from build123d import *

# Parameters (mm, degrees)
BOSS_EXTRUDE1_DEPTH     = 4
SKETCH3_W               = 9
SKETCH3_H               = 19
SKETCH3_W_2             = 19
SKETCH3_H_2             = 9
BOSS_EXTRUDE2_DEPTH     = 1
CHAMFER1_SIZE           = 1
CUT_EXTRUDE1_DEPTH      = 86
CUT_EXTRUDE1_DEPTH_BACK = 86
SKETCH2_R               = 2.5


with BuildPart() as part:
    # Sketch1 → Boss-Extrude1 (new body)
    with BuildSketch(Plane(origin=(0, 0, 0), x_dir=(1, 0, 0), z_dir=(0, 1, 0))):
        Polygon((0, 0), (0, 60), (20, 60), (60, 20), (60, 0), align=None)
    extrude(amount=BOSS_EXTRUDE1_DEPTH)

    # Sketch3 → Boss-Extrude2 (add)
    with BuildSketch(Plane(origin=(0, 4, 0), x_dir=(1, 0, 0), z_dir=(0, 1, 0))):
        with Locations((10, 50.5)):
            Rectangle(SKETCH3_W, SKETCH3_H)
        with Locations((50.5, 10)):
            Rectangle(SKETCH3_W_2, SKETCH3_H_2)
    extrude(amount=BOSS_EXTRUDE2_DEPTH)

    # Chamfer1
    chamfer1_edges = [part.edges().sort_by_distance(p)[0] for p in [
        (50.5, 5, -14.5),
        (50.5, 5, -5.5),
        (14.5, 5, -50.5),
        (5.5, 5, -50.5),
    ]]
    chamfer(chamfer1_edges, length=CHAMFER1_SIZE - 0.0001)  # a hair under: the kernel refuses the full size

    # Sketch2 → Cut-Extrude1 (cut, two sides: drawn at the far end of the back side and taken through both)
    with BuildSketch(Plane.XZ.offset(-CUT_EXTRUDE1_DEPTH_BACK)):
        with Locations(Location((50, -10, 0), (0, 0, 270))):
            Circle(SKETCH2_R)
        with Locations(Location((30, -10, 0), (0, 0, 90))):
            Circle(SKETCH2_R)
        with Locations(Location((10, -10, 0), (0, 0, 90))):
            Circle(SKETCH2_R)
        with Locations(Location((10, -30, 0), (0, 0, 90))):
            Circle(SKETCH2_R)
        with Locations(Location((10, -50, 0), (0, 0, 270))):
            Circle(SKETCH2_R)
        with BuildLine():
            Line((48.292989119, -21.707106781), (38.207130756, -31.792965144))
            ThreePointArc((38.207130756, -31.792965144), (37.500023975, -32.085858363), (36.792917194, -31.792965144))
            Line((36.792917194, -31.792965144), (26.707058831, -21.707106781))
            ThreePointArc((26.707058831, -21.707106781), (26.49028608, -20.617316568), (27.414165612, -20))
            Line((27.414165612, -20), (47.585882338, -20))
            ThreePointArc((47.585882338, -20), (48.509761871, -20.617316568), (48.292989119, -21.707106781))
        make_face()
        with BuildLine():
            Line((31.792965144, -36.792917194), (21.707106781, -26.707058831))
            ThreePointArc((21.707106781, -26.707058831), (20.617316568, -26.49028608), (20, -27.414165612))
            Line((20, -27.414165612), (20, -47.585882338))
            ThreePointArc((20, -47.585882338), (20.617316568, -48.509761871), (21.707106781, -48.292989119))
            Line((21.707106781, -48.292989119), (31.792965144, -38.207130756))
            ThreePointArc((31.792965144, -38.207130756), (32.085858363, -37.500023975), (31.792965144, -36.792917194))
        make_face()
    extrude(amount=CUT_EXTRUDE1_DEPTH + CUT_EXTRUDE1_DEPTH_BACK, mode=Mode.SUBTRACT)


solid = part.part
CAD build for the part. Positions are in the model's coordinates, mm. A direction names the side the tool comes from. Coordinates: 2 decimals unless noted, no trailing zeros. Write each loop counter-clockwise with the first axis right and the second up, starting at its lowest first coordinate (ties: lowest second). Pieces come first, ordered by that corner, then holes. Notation, with made-up numbers: (-18, 5.5) - (11, 5.5) arc R18 ccw to (11, 17.5) - close; hole circle Ø5 at (20.25, 53.25). An arc over 180 degrees is marked (long way). Use a Markdown table: item, result. Add a question column.
Item 1: 3-axis set-ups, long thin cutter, end or side, ignore diameter. For faces 4 (the face through (32, 2, -27)), 5 (the face through (0, 2, -30)): which of +Z, -Z, +X, -X, +Y, -Y reach the whole face in a straight line?
Item 2: Band-saw the part on C-C, the plane x = 10. Give the cut face in (y, z), and give its area (3 significant figures).
Item 3: Band-saw the part on B-B, the plane z = -10. Give the cut face in (x, y), and give its area (3 significant figures).
Item 4: Flat gauge pins, fed straight in: pin 1 (5 mm diameter, centred on x = 28.5, z = -9.5, fed in from +Y); pin 2 (3 mm diameter, centred on x = 33, y = 2.5, fed in from -Z); pin 3 (0.5 mm diameter, centred on y = 4.5, z = -8, fed in from -X). Where does each tip first touch, or does it go through?
Item 5: Mould opens along Z. For faces 1 (the face through (40, 2, -40)), 2 (the face through (30, 2, 0)), 3 (the face through (37.511, 2.028, -32.086)) say: pulls with the +Z half, pulls with the -Z half, needs draft (parallel to the pull), parting line crosses it, or undercut.
Item 6: Drill centre lines: L1, parallel to X at y = 2.4, z = -10; L2, parallel to X at y = 2.35, z = -30; L3, parallel to Z at x = 28.5, y = 1.5. Where is each one in solid material? Low to high. Write a range as from..to.
Item 7: Band-saw the part on D-D, the plane y = 2.05. Give the cut face in (x, z), and give its area (3 significant figures).
Numbers:
| question | item | result |
|---|---|---|
| 1 | face 4 | +Y, -Y |
| 1 | face 5 | +Z, -Z, -X, +Y, -Y |
| 2 | outline | (0, -60) - (5, -60) - (5, -52.5) - (0, -52.5) - close; (0, -47.5) - (5, -47.5) - (5, -41) - (4, -41) - (4, -32.5) - (0, -32.5) - close; (0, -27.5) - (4, -27.5) - (4, -12.5) - (0, -12.5) - close; (0, -7.5) - (4, -7.5) - (4, 0) - (0, 0) - close |
| 2 | area | 194 mm2 |
| 3 | outline | (0, 0) - (7.5, 0) - (7.5, 4) - (0, 4) - close; (12.5, 0) - (27.5, 0) - (27.5, 4) - (12.5, 4) - close; (32.5, 0) - (47.5, 0) - (47.5, 5) - (41, 5) - (41, 4) - (32.5, 4) - close; (52.5, 0) - (60, 0) - (60, 5) - (52.5, 5) - close |
| 3 | area | 194 mm2 |
| 4 | pin 1 | y = 4 |
| 4 | pin 2 | z = -48.5 |
| 4 | pin 3 | x = 41 |
| 5 | face 1 | pulls with the -Z half |
| 5 | face 2 | pulls with the +Z half |
| 5 | face 3 | undercut |
| 6 | L1 | 0..7.5, 12.5..27.5, 32.5..47.5, 52.5..60 |
| 6 | L2 | 0..7.5, 12.5..20, 25..35, 40..50 |
| 6 | L3 | -51.5..-41.5, -33.5..-23.5, -20..-12, -8..0 |
| 7 | outline | (0, -60) - (20, -60) - (60, -20) - (60, 0) - (0, 0) - close; hole circle Ø5 at (10, -50); hole circle Ø5 at (10, -30); hole circle Ø5 at (10, -10); hole (20, -47.59) arc R1 ccw to (21.71, -48.29) - (31.79, -38.21) arc R1 ccw to (31.79, -36.79) - (21.71, -26.71) arc R1 ccw to (20, -27.41) - close; hole (26.71, -21.71) - (36.79, -31.79) arc R1 ccw to (38.21, -31.79) - (48.29, -21.71) arc R1 ccw to (47.59, -20) - (27.41, -20) arc R1 ccw to start; hole circle Ø5 at (30, -10); hole circle Ø5 at (50, -10) |
| 7 | area | 2,390 mm2 |
